from build123d import *

# Parameters (mm, degrees)
F1_DEPTH = 1.27


with BuildPart() as f1:
    # F0 (on Top) → F1 (new body)
    with BuildSketch(Plane.XY):
        with BuildLine():
            ThreePointArc((-2.882069, 17.221197), (-3.590437, 19.489788), (-4.770173, 21.55292))
            ThreePointArc((-4.770173, 21.55292), (-9.848493, 24.526917), (-14.97957, 21.644898))
            ThreePointArc((-14.97957, 21.644898), (-17.126716, 18.50464), (-18.658631, 15.022587))
            ThreePointArc((-18.658631, 15.022587), (-19.628382, 12.011872), (-20.028973, 8.874301))
            ThreePointArc((-20.028973, 8.874301), (-20.243217, 6.190879), (-20.028973, 3.507457))
            ThreePointArc((-20.028973, 3.507457), (-19.536147, 0.849985), (-18.824216, -1.757349))
            ThreePointArc((-18.824216, -1.757349), (-18.221226, -4.422973), (-17.734695, -7.112292))
            ThreePointArc((-17.734695, -7.112292), (-17.5082, -9.985099), (-17.261155, -12.856212))
            ThreePointArc((-17.261155, -12.856212), (-17.121014, -15.18523), (-16.90908, -17.508816))
            ThreePointArc((-16.90908, -17.508816), (-16.723027, -19.570727), (-16.204746, -21.575091))
            ThreePointArc((-16.204746, -21.575091), (-14.961127, -24.553308), (-12.275964, -26.343912))
            ThreePointArc((-12.275964, -26.343912), (-8.705685, -26.680746), (-5.55828, -24.961971))
            ThreePointArc((-5.55828, -24.961971), (-3.915633, -21.699123), (-3.790411, -18.048262))
            ThreePointArc((-3.790411, -18.048262), (-4.280415, -12.974763), (-4.946626, -7.921382))
            ThreePointArc((-4.946626, -7.921382), (-5.055093, -2.952952), (-4.197766, 1.942152))
            ThreePointArc((-4.197766, 1.942152), (-3.012476, 5.886456), (-2.503398, 9.973422))
            ThreePointArc((-2.503398, 9.973422), (-2.409428, 13.612111), (-2.882069, 17.221197))
        make_face()
    extrude(amount=F1_DEPTH)


solid = f1.part
The listing builds one solid part. Answer for the finished solid, in the listing's coordinates (mm). Give positions to 0.01 mm unless a question says otherwise; leave off trailing zeros. Write each loop counter-clockwise with the first axis right and the second up, starting at its lowest first coordinate (ties: lowest second). Pieces come first, ordered by that corner, then holes. Notation, with made-up numbers: (-12.5, 61) - (11.5, 61) arc R33 cw to (11.5, 93) - close; hole circle Ø7 at (18, 23.25). An arc over 180 degrees is marked (long way). One line per question, with ' | ' between items. Start each with the question number.
1. Straight lines are drawn through the part: line 1 (Y direction, x = -9.75, z = 1.1); line 2 (Y direction, x = -8.25, z = 0.7); line 3 (X direction, y = 19.5, z = 0.15). For each, find the intervals that lie inside material, in ascending order.
2. Determine the mould class of faces 1 (the face through (-2.407, 13.561, 0.626)), 2 (the face through (-19.545, 0.887, 0.626)), 3 (the face through (-9.762, 24.526, 0.626)), 4 (the face through (-3.024, 5.83, 0.626)) for opening direction Y: +Y half, -Y half, draft (parallel to the pull), parting line (faces both ways), or undercut.
3. Section C-C, the plane y = -3 is taken. Determine the outline of the cut face in (x, z), then the cut area to 3 significant figures.
4. Section B-B, the plane x = -13 is taken. Determine the outline of the cut face in (y, z), then the cut area to 3 significant figures.
5. Section A-A, the plane z = 0.9 is taken. Determine the outline of the cut face in (x, y).
Result:
1) line 1: y = -26.8 to 24.53 | line 2: y = -26.57 to 24.29 | line 3: x = -16.54 to -3.59
2) face 1: parting line | face 2: -Y half | face 3: +Y half | face 4: undercut
3) outline: (-18.53, 0) - (-5.06, 0) - (-5.06, 1.27) - (-18.53, 1.27) - close | area: 17.1 mm2
4) outline: (-26.07, 0) - (23.65, 0) - (23.65, 1.27) - (-26.07, 1.27) - close | area: 63.1 mm2
5) outline: (-20.03, 3.51) arc R32.5 ccw to (-18.82, -1.76) arc R62.85 cw to (-17.73, -7.11) arc R402.74 ccw to (-17.26, -12.86) arc R75.61 ccw to (-16.91, -17.51) arc R12.71 ccw to (-16.2, -21.58) arc R5.58 ccw to (-12.28, -26.34) arc R6.13 ccw to (-5.56, -24.96) arc R8.52 ccw to (-3.79, -18.05) arc R146.49 ccw to (-4.95, -7.92) arc R25.5 cw to (-4.2, 1.94) arc R24.54 ccw to (-2.5, 9.97) arc R23.35 ccw to (-2.88, 17.22) arc R10.98 ccw to (-4.77, 21.55) arc R5.91 ccw to (-14.98, 21.64) arc R20.56 ccw to (-18.66, 15.02) arc R17.16 ccw to (-20.03, 8.87) arc R16.91 ccw to start
